Here's how the part is built. I have some questions about the finished solid (model axes, mm). Face numbers are marked on the shaded views. A direction names the side the tool comes from. Coordinates: 2 decimals unless noted, no trailing zeros. Write each loop counter-clockwise with the first axis right and the second up, starting at its lowest first coordinate (ties: lowest second). Pieces come first, ordered by that corner, then holes. Notation, with made-up numbers: (76.5, 40) - (105.5, 40) arc R34 ccw to (105.5, 75) - close; hole circle Ø1 at (82, 84). An arc over 180 degrees is marked (long way). Answer in a Markdown table with one row per item. Add a question column.
Item 1: Which directions (+Z, -Z, +X, -X, +Y, -Y) give clear straight access to the entire face, cutting with the end or side of a thin tool? Please do the marked faces 1, 2 and 3.
Item 2: I'm going to push flat-ended pins straight in: pin 1 (1.5 mm diameter, centred on x = -0.5, z = -15, fed in from -Y); pin 2 (1.5 mm diameter, centred on y = 15.5, z = 14, fed in from -X); pin 3 (5 mm diameter, centred on x = 4, z = -9.5, fed in from -Y). Where does each tip first touch, or does it pass through?
Item 3: Imagine slicing it at D-D (y = 13.5). Please give me the cut outline in (x, z).
Item 4: Imagine slicing it at B-B (z = 0). Please give me the cut outline in (x, y).
Item 5: Imagine slicing it at C-C (y = 1.5). Please give me the cut outline in (x, z), plus the area to 3 significant figures.
Item 6: If I drill on probe 1 along X at (y, z) = (3.85, 0); probe 2 along Y at (x, z) = (-11.5, -1); probe 3 along X at (y, z) = (-15, 3), over which ranges is the centre line in solid material (lowest first)? Write a range as from..to.
Item 7: Imagine slicing it at A-A (x = 0). Please give me the cut outline in (y, z), plus the area to 3 significant figures.
from build123d import *

# Parameters (mm, degrees)
SKETCH1_R           = 18
BOSS_EXTRUDE1_DEPTH = 40
SKETCH2_R           = 1.5
CUT_EXTRUDE1_DEPTH  = 5
CIRPATTERN1_COUNT   = 4
SKETCH3_R           = 11
BOSS_EXTRUDE2_DEPTH = 3
SKETCH4_R           = 4
BOSS_EXTRUDE3_DEPTH = 17
CUT_EXTRUDE2_START  = -15
CUT_EXTRUDE2_DEPTH  = 15


with BuildPart() as part:
    # Sketch1 → Boss-Extrude1 (new body)
    with BuildSketch(Plane(origin=(0, 0, 0), x_dir=(1, 0, 0), z_dir=(0, 1, 0))):
        with Locations(Location((0, 0, 0), (0, 0, 270))):
            Circle(SKETCH1_R)
    extrude(amount=BOSS_EXTRUDE1_DEPTH)

    # Sketch2 → Cut-Extrude1 (cut)
    with BuildSketch(Plane.XZ):
        with Locations(Location((-15, 0, 0), (0, 0, 270))):
            Circle(SKETCH2_R)
    cut_extrude1 = extrude(amount=-CUT_EXTRUDE1_DEPTH, mode=Mode.SUBTRACT)

    # CirPattern1: Cut-Extrude1 ×4 about axis
    cirpattern1_axis = Axis((0, 0, 0), (0, 1, 0))
    for i in range(1, CIRPATTERN1_COUNT):
        add(cut_extrude1.rotate(cirpattern1_axis, i * 360 / CIRPATTERN1_COUNT), mode=Mode.SUBTRACT)

    # Sketch3 → Boss-Extrude2 (add)
    with BuildSketch(Plane.XZ):
        with Locations(Location((0, 0, 0), (0, 0, 90))):
            Circle(SKETCH3_R)
    extrude(amount=BOSS_EXTRUDE2_DEPTH)

    # Sketch4 → Boss-Extrude3 (add)
    with BuildSketch(Plane.XZ.offset(3)):
        with Locations(Location((0, 0, 0), (0, 0, 270))):
            Circle(SKETCH4_R)
    extrude(amount=BOSS_EXTRUDE3_DEPTH)

    # Sketch5 → Cut-Extrude2 (cut)
    with BuildSketch(Plane.XZ.offset(20).offset(CUT_EXTRUDE2_START)):
        with BuildLine():
            Line((-2.645751311, -3), (2.645751311, -3))
            ThreePointArc((2.645751311, -3), (0, -4), (-2.645751311, -3))
        make_face()
    extrude(amount=CUT_EXTRUDE2_DEPTH, mode=Mode.SUBTRACT)


solid = part.part
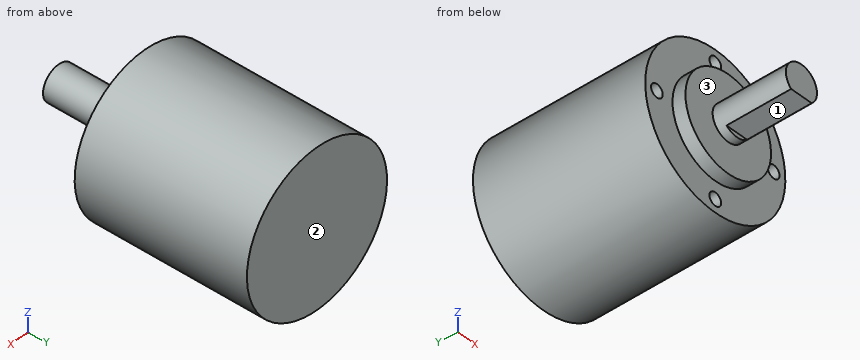
Here are the results:
| question | item | result |
|---|---|---|
| 1 | face 1 | -Z, +X, -X, -Y |
| 1 | face 2 | +Z, -Z, +X, -X, +Y |
| 1 | face 3 | -Y |
| 2 | pin 1 | stops at y = 5 |
| 2 | pin 2 | stops at x = -12.18 |
| 2 | pin 3 | stops at y = -3 |
| 3 | outline | circle Ø36 at (0, 0) |
| 4 | outline | (-18, 0) - (-16.5, 0) - (-16.5, 5) - (-13.5, 5) - (-13.5, 0) - (-11, 0) - (-11, -3) - (-4, -3) - (-4, -20) - (4, -20) - (4, -3) - (11, -3) - (11, 0) - (13.5, 0) - (13.5, 5) - (16.5, 5) - (16.5, 0) - (18, 0) - (18, 40) - (-18, 40) - close |
| 5 | outline | circle Ø36 at (0, 0); hole circle Ø3 at (-15, 0); hole circle Ø3 at (0, -15); hole circle Ø3 at (0, 15); hole circle Ø3 at (15, 0) |
| 5 | area | 990 mm2 |
| 6 | probe 1 | x = -18..-16.5, -13.5..13.5, 16.5..18 |
| 6 | probe 2 | y = 0..40 |
| 6 | probe 3 | x = -2.65..2.65 |
| 7 | outline | (-20, -3) - (-5, -3) - (-5, -4) - (-3, -4) - (-3, -11) - (0, -11) - (0, -13.5) - (5, -13.5) - (5, -16.5) - (0, -16.5) - (0, -18) - (40, -18) - (40, 18) - (0, 18) - (0, 16.5) - (5, 16.5) - (5, 13.5) - (0, 13.5) - (0, 11) - (-3, 11) - (-3, 4) - (-20, 4) - close |
| 7 | area | 1,600 mm2 |
